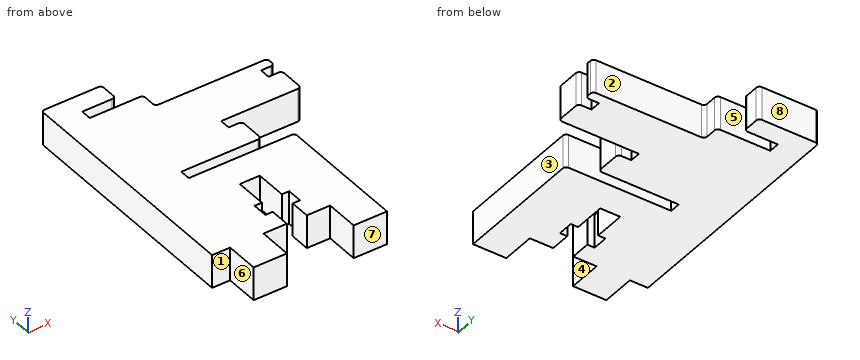
from build123d import *

# Parameters (mm, degrees)
BOSS_EXTRUDE1_DEPTH = 5
FILLET3_R           = 0.5


with BuildPart() as part:
    # Sketch1 → Boss-Extrude1 (new body)
    with BuildSketch(Plane.XY):
        Polygon((4.1, 19.6), (4.1, 21.2), (16.1, 21.2), (16.1, 25.3), (14.1, 25.3), (14.1, 26.9), (26.1, 26.9), (26.1, 31), (24.1, 31), (24.1, 32.6), (26.1, 32.6), (26.1, 34.1), (9.3, 34.1), (9.3, 36.7), (1.3, 36.7), (1.3, 38.3), (6.3, 38.3), (6.3, 41.3), (-2.7, 41.3), (-2.7, 5), (0, 5), (0, 0), (5, 0), (5, 5), (8.5, 5), (8.5, 8), (7.4, 8), (7.4, 10.3), (8.5, 10.3), (8.5, 15), (11.5, 15), (11.5, 10.3), (12.6, 10.3), (12.6, 8), (11.5, 8), (11.5, 5), (15, 5), (15, 0), (20, 0), (20, 5), (20, 19.6), align=None)
    extrude(amount=BOSS_EXTRUDE1_DEPTH)

    # Fillet3
    fillet3_edges = [part.edges().sort_by_distance(p)[0] for p in [
        (-2.7, 41.3, 2.5),
        (6.3, 41.3, 2.5),
        (6.3, 38.3, 2.5),
        (9.3, 36.7, 2.5),
        (9.3, 34.1, 2.5),
        (26.1, 34.1, 2.5),
        (26.1, 32.6, 2.5),
        (26.1, 31, 2.5),
        (26.1, 26.9, 2.5),
        (16.1, 25.3, 2.5),
        (16.1, 21.2, 2.5),
        (20, 19.6, 2.5),
    ]]
    fillet(fillet3_edges, radius=FILLET3_R)


solid = part.part
The listing builds one solid part. Answer for the finished solid, in the listing's coordinates (mm). Face numbers are marked on the shaded views. A direction names the side the tool comes from. Coordinates: 2 decimals unless noted, no trailing zeros. Order: outer loops, then holes, each group sorted by start corner. A loop starts at its lowest first (then second) coordinate and runs counter-clockwise, first axis right, second up.
Q1. A cutting plane is placed at D-D, the plane x = 22. Write down the section's boundary in (y, z).
Q2. A cutting plane is placed at C-C, the plane y = 26. Write down the section's boundary in (x, z), and give its area (3 significant figures).
Q3. A cutting plane is placed at B-B, the plane y = 12.5. Write down the section's boundary in (x, z), and give its area (3 significant figures).
Q4. Given P1, Ø5, axis at x = 14, y = 18, coming from the -Z side; P2, Ø1.8, axis at y = 20, z = 2.5, coming from the +X side; P3, Ø0.8, axis at y = 31.5, z = 2.5, coming from the +X side; P4, Ø2.5, axis at y = 1.5, z = 2.5, coming from the -X side, each flat-ended and moving along its own axis, determine where each tip first touches the part or whether it passes through.
Q5. A cutting plane is placed at A-A, the plane x = 18.5. Write down the section's boundary in (y, z), and give its area (3 significant figures).
Q6. Which of the six approach directions +Z, -Z, +X, -X, +Y, -Y give full straight-line access (tool end or side, diameter ignored) to the marked faces 1, 2, 3 and 4?
Q7. Consider line 1 (Y direction, x = 8, z = 2.3); line 2 (Y direction, x = 14, z = 2.05); line 3 (Y direction, x = 16.5, z = 4.45). Determine where each line is inside the solid, lowest interval first.
Q8. For a pull along Y with two mould halves and no side action, classify the marked faces 5, 6, 7 and 8 as pulls with the +Y half, pulls with the -Y half, needs draft (parallel to the pull), parting line crosses it, or undercut.
Answers follow:
1. outline: (26.9, 0) - (34.1, 0) - (34.1, 5) - (26.9, 5) - close
2. outline: (-2.7, 0) - (14.1, 0) - (14.1, 5) - (-2.7, 5) - close
2. area: 84.0 mm2
3. outline: (-2.7, 0) - (8.5, 0) - (8.5, 5) - (-2.7, 5) - close; (11.5, 0) - (20, 0) - (20, 5) - (11.5, 5) - close
3. area: 98.5 mm2
4. P1: stops at z = 0
4. P2: stops at x = 20
4. P3: stops at x = 24.1
4. P4: stops at x = 0
5. outline: (0, 0) - (19.6, 0) - (19.6, 5) - (0, 5) - close; (26.9, 0) - (34.1, 0) - (34.1, 5) - (26.9, 5) - close
5. area: 134 mm2
6. face 1: +Z, -Z, -X, -Y
6. face 2: +Z, -Z, +X, +Y
6. face 3: +Z, -Z, +X, -Y
6. face 4: +Z, -Z, -Y
7. line 1: y = 5 to 8, 10.3 to 19.6, 21.2 to 36.7
7. line 2: y = 5 to 19.6, 21.2 to 34.1
7. line 3: y = 0 to 19.6, 26.9 to 34.1
8. face 5: undercut
8. face 6: needs draft
8. face 7: pulls with the -Y half
8. face 8: pulls with the +Y half
